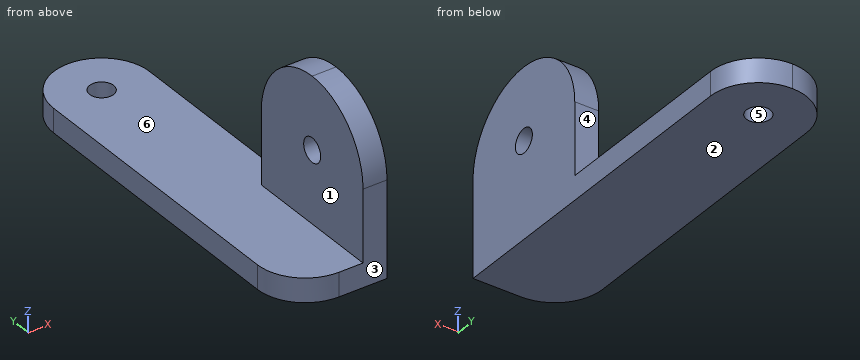
from build123d import *

# Parameters (mm, degrees)
ESQUISSE1_W             = 20
ESQUISSE1_H             = 80
BOSS_EXTRU_1_DEPTH      = 5
ESQUISSE2_R             = 2.5
ENL_V_MAT_EXTRU_1_DEPTH = 5
ESQUISSE3_W             = 5
ESQUISSE3_H             = 30
BOSS_EXTRU_2_DEPTH      = 30
ESQUISSE4_R             = 2.5
ENL_V_MAT_EXTRU_2_DEPTH = 30
CONG_1_R                = 15
CONG_2_R                = 10


with BuildPart() as part:
    # Esquisse1 → Boss.-Extru.1 (new body)
    with BuildSketch(Plane.XY):
        with Locations((-7.390726734, -27.034940778)):
            Rectangle(ESQUISSE1_W, ESQUISSE1_H)
    extrude(amount=BOSS_EXTRU_1_DEPTH)

    # Esquisse2 → Enlèv. mat.-Extru.1 (cut)
    with BuildSketch(Plane.XY.offset(5)):
        with Locations((-7.390726734, 2.965059222)):
            Circle(ESQUISSE2_R)
    extrude(amount=-ENL_V_MAT_EXTRU_1_DEPTH, mode=Mode.SUBTRACT)

    # Esquisse3 → Boss.-Extru.2 (add)
    with BuildSketch(Plane.XY.offset(5)):
        with Locations((0.109273266, -52.034940778)):
            Rectangle(ESQUISSE3_W, ESQUISSE3_H)
    extrude(amount=BOSS_EXTRU_2_DEPTH)

    # Esquisse4 → Enlèv. mat.-Extru.2 (cut)
    with BuildSketch(Plane(origin=(2.609273266, 0, 0), x_dir=(0, 0, -1), z_dir=(1, 0, 0))):
        with Locations(Location((-20, -52.034940778, 0), (0, 0, 90))):
            Circle(ESQUISSE4_R)
    extrude(amount=-ENL_V_MAT_EXTRU_2_DEPTH, mode=Mode.SUBTRACT)

    # Congé1
    cong_1_edges = [part.edges().sort_by_distance(p)[0] for p in [
        (0.109273266, -67.034940778, 35),
        (0.109273266, -37.034940778, 35),
    ]]
    fillet(cong_1_edges, radius=CONG_1_R - 0.0001)  # a hair under: the kernel refuses the full size

    # Congé2
    cong_2_edges = [part.edges().sort_by_distance(p)[0] for p in [
        (-17.390726734, -67.034940778, 2.5),
        (2.609273266, 12.965059222, 2.5),
        (-17.390726734, 12.965059222, 2.5),
    ]]
    fillet(cong_2_edges, radius=CONG_2_R - 0.0001)  # a hair under: the kernel refuses the full size


solid = part.part
Verification items for the finished model (mm, model axes). Face numbers are marked on the shaded views. A direction names the side the tool comes from. Round coordinates to 2 decimals unless told otherwise and drop trailing zeros. Write each loop counter-clockwise with the first axis right and the second up, starting at its lowest first coordinate (ties: lowest second). Pieces come first, ordered by that corner, then holes.
(1) Material ranges on line 1 (Z direction, x = -13.5, y = -14); line 2 (Y direction, x = 0.25, z = 11); line 3 (X direction, y = -43.5, z = 31), recorded low to high.
Returned:
line 1: z = 0 to 5
line 2: y = -67.03 to -37.03
line 3: x = -2.39 to 2.61
(2) Depth check by flat-ended pin: pin 1 Ø10 at (y, z) = (-52, 29.5) entering from -X; pin 2 Ø12 at (y, z) = (-32, 6) entering from -X; pin 3 Ø5.5 at (x, z) = (-0.5, 11.5) entering from +Y; pin 4 Ø6 at (x, y) = (-12.5, -34) entering from +Z. Enter the tip coordinate at first touch or a pass-through.
Returned:
pin 1: stops at x = -2.39
pin 2: stops at x = -17.39
pin 3: stops at y = -37.03
pin 4: stops at z = 5
(3) Section check C-C (z = 8.5). Enter the section's corners in (x, y), plus the area to 3 significant figures.
Returned:
outline: (-2.39, -67.03) - (2.61, -67.03) - (2.61, -37.03) - (-2.39, -37.03) - close
area: 150 mm2
(4) Access from +Z, -Z, +X, -X, +Y, -Y to the whole of each face (thin tool, end or side, straight path). Record for the marked faces 1 and 2.
Returned:
face 1: +Z, -X, +Y, -Y
face 2: -Z, +X, -X, +Y, -Y
(5) Mould release check, pull along Y, two halves, no side actions. Record for the marked faces 3, 4, 5 and 6: pulls with the +Y half, pulls with the -Y half, needs draft (parallel to the pull), parting line crosses it, or undercut.
Returned:
face 3: pulls with the -Y half
face 4: pulls with the +Y half
face 5: undercut
face 6: needs draft
(6) Section check B-B (y = -29.5). Enter the section's corners in (x, z).
Returned:
outline: (-17.39, 0) - (2.61, 0) - (2.61, 5) - (-17.39, 5) - close
(7) Section check D-D (y = -38.5). Enter the section's corners in (x, z), plus the area to 3 significant figures.
Returned:
outline: (-17.39, 0) - (2.61, 0) - (2.61, 26.47) - (-2.39, 26.47) - (-2.39, 5) - (-17.39, 5) - close
area: 207 mm2
(8) Section check A-A (z = 21). Enter the section's corners in (x, y).
Returned:
outline: (-2.39, -67) - (2.61, -67) - (2.61, -54.33) - (-2.39, -54.33) - close; (-2.39, -49.74) - (2.61, -49.74) - (2.61, -37.07) - (-2.39, -37.07) - close
